Here's how the part is built. I have some questions about the finished solid (model axes, mm). A direction names the side the tool comes from. Coordinates: 2 decimals unless noted, no trailing zeros. Order: outer loops, then holes, each group sorted by start corner. A loop starts at its lowest first (then second) coordinate and runs counter-clockwise, first axis right, second up. Notation, with made-up numbers: (34.5, -13) - (88.5, -13) arc R29 cw to (88.5, 24) - close; hole circle Ø6 at (50, 16.5). An arc over 180 degrees is marked (long way). Answer in a Markdown table with one row per item. Add a question column.
Item 1: On a 3-axis mill with a long thin cutter (end or side, diameter ignored), from which of +Z, -Z, +X, -X, +Y, -Y can I reach the whole of each face in a straight line? I mean faces 4 (the flat face through (-7.982, -3, 1)), 5 (the cylindrical face through (-12.96, 5.18, 4.46)). Say none if no direction works.
Item 2: I want a section at C-C (y = -1.75). Please give me the cut outline in (x, z).
Item 3: Thinking about a two-plate mould opening in X: for faces 1 (the flat face through (-15.982, -3, 1)), 2 (the cylindrical face through (-10.55, -4.1, 0.76)), 3 (the flat face through (-12.04, -2.88, 1.5)), which applies, +X half, -X half, draft (parallel to the pull), parting line (faces both ways), or undercut?
Item 4: If I drill on line 1 along Z through (x, y) = (-11.5, 4.25); line 2 along Y through (x, z) = (-11.5, 3.75); line 3 along X through (y, z) = (-5.5, 1.25) (1 decimal), over which ranges is the centre line in solid material (lowest first)? Write a range as from..to.
Item 5: I want a section at A-A (x = -13). Please give me the cut outline in (y, z).
Item 6: I want a section at B-B (z = 4.5). Please give me the cut outline in (x, y).
```python
from build123d import *

# Parameters (mm, degrees)
SKETCH1_W           = 8
SKETCH1_H           = 24
BOSS_EXTRUDE1_DEPTH = 1.5
SKETCH2_R           = 1.5
CUT_EXTRUDE1_DEPTH  = 2.5
SKETCH3_R           = 1.25
BOSS_EXTRUDE3_DEPTH = 6


with BuildPart() as part:
    # Sketch1 → Boss-Extrude1 (new body)
    with BuildSketch(Plane.XY):
        with Locations((-11.98249453, -3.04595186)):
            Rectangle(SKETCH1_W, SKETCH1_H)
    extrude(amount=BOSS_EXTRUDE1_DEPTH)

    # Sketch2 → Cut-Extrude1 (cut, through all)
    with BuildSketch(Plane.XY.offset(1.5)):
        with Locations((-11.98249453, -4.54595186)):
            Circle(SKETCH2_R)
    extrude(amount=-CUT_EXTRUDE1_DEPTH, mode=Mode.SUBTRACT)

    # Sketch3 → Boss-Extrude3 (add)
    with BuildSketch(Plane.XY.offset(1.5)):
        with Locations((-11.965684197, 5.940322957)):
            Circle(SKETCH3_R)
        with Locations((-11.965684197, 1.940322957)):
            Circle(SKETCH3_R)
    extrude(amount=BOSS_EXTRUDE3_DEPTH)


solid = part.part
```
Values follow:
| question | item | result |
|---|---|---|
| 1 | face 4 | +Z, -Z, +X, +Y, -Y |
| 1 | face 5 | +Z |
| 2 | outline | (-15.98, 0) - (-7.98, 0) - (-7.98, 1.5) - (-15.98, 1.5) - close |
| 3 | face 1 | -X half |
| 3 | face 2 | undercut |
| 3 | face 3 | draft |
| 4 | line 1 | z = 0..1.5 |
| 4 | line 2 | y = 0.78..3.1, 4.78..7.1 |
| 4 | line 3 | x = -16..-13.1, -10.8..-8 |
| 5 | outline | (-15.05, 0) - (-5.65, 0) - (-5.65, 1.5) - (-15.05, 1.5) - close; (-3.44, 0) - (8.95, 0) - (8.95, 1.5) - (6.64, 1.5) - (6.64, 7.5) - (5.24, 7.5) - (5.24, 1.5) - (2.64, 1.5) - (2.64, 7.5) - (1.24, 7.5) - (1.24, 1.5) - (-3.44, 1.5) - close |
| 6 | outline | circle Ø2.5 at (-11.97, 1.94); circle Ø2.5 at (-11.97, 5.94) |
